CAD build for the part. Positions are in the model's coordinates, mm. Face numbers are marked on the shaded views. A direction names the side the tool comes from. Give positions to 0.01 mm unless a question says otherwise; leave off trailing zeros. Order: outer loops, then holes, each group sorted by start corner. A loop starts at its lowest first (then second) coordinate and runs counter-clockwise, first axis right, second up.
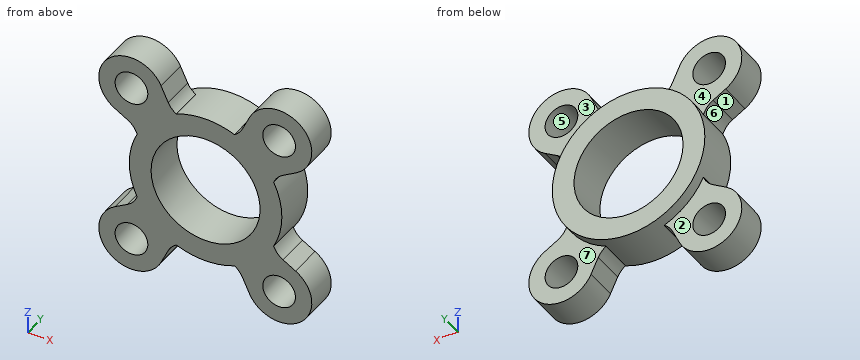
Autodesk Inventor part; units mm, degrees
ref_plane "YZ Plane" through (0, 0, 0) normal (1, 0, 0) x (0, 1, 0)
ref_plane "XZ Plane" through (0, 0, 0) normal (0, 1, 0) x (-1, 0, 0)
ref_plane "XY Plane" through (0, 0, 0) normal (0, 0, 1) x (1, 0, 0)
sketch "Эскиз1" plane through (0, 0, 0) normal (0, 1, 0) x (-1, 0, 0)
  circle A0 centre (-0.0254, 0) radius 7
  circle A1 centre (-7.0254, 6.889) radius 1.5
  circle A2 centre (6.7752, 7.433) radius 1.5
  circle A3 centre (6.9746, -7.0215) radius 1.5
  circle A4 centre (-7.0254, -7.0215) radius 1.5
  circle A5 centre (-0.0254, 0) radius 5
  line L0 (0, 0) -> (0, 8.1981) construction
  line L1 (-0.0254, 0) -> (8.1589, 0) construction
  circle A6 centre (6.7752, 7.433) radius 3
  line L2 (4.0592, 8.7071) -> (3.4025, 7.3072)
  line L3 (8.2851, 4.8407) -> (7.1407, 4.1741)
  line L4 (0.7424, 6.346) -> (0.4551, 6.4808)
  arc A7 (0.7424, 6.346) -> (3.4025, 7.3072) centre (1.5918, 8.1566) ccw
  line L5 (5.7914, 2.5169) -> (6.4192, 1.4392)
  arc A8 (7.1407, 4.1741) -> (6.4192, 1.4392) centre (8.1474, 2.4459) ccw
  point P0 (-10.336, -7.0215)
  point P1 (-9.1433, 6.8618)
  point P2 (6.9746, 10.1261)
  point P3 (2.6587, 6.4649)
  point P4 (6.2546, 3.0921)
  dimension "d0" = 14
  dimension "d1" = 3
  dimension "d2" = 3
  dimension "d3" = 3
  dimension "d4" = 3
  dimension "d5" = 10
  dimension "d6" = 6
  dimension "d7" = 2
  dimension "d8" = 2
extrude "Выдавливание1" add sketch "Эскиз1" along normal blind 4 contours A0
extrude "Выдавливание2" add sketch "Эскиз1" along normal blind 3 contours A0 A7 L2 A6 L3 A8 | A6
mirror "Зеркальное отражение1" about plane through (0, 0, 0) normal (1, 0, 0) of "Выдавливание2"
mirror "Зеркальное отражение2" about plane through (0, 0, 0) normal (0, 0, 1) of "Выдавливание2", "Зеркальное отражение1"
properties part number "крепление подшипника_1"
1. Saw through at B-B on x = 5.75. Give the cut face in (y, z).
2. Saw through at C-C on y = 2.45. State how many separate pieces and enclosed holes the cut face has, plus the area to 3 significant figures.
3. Saw through at D-D on x = -3. Give the cut face in (y, z), plus the area to 3 significant figures.
4. Pin check, flat tips, straight feed: P1, Ø1.5, axis at y = 1.5, z = 4.5, coming from the -X side; P2, Ø5, axis at x = 6.78, z = -7.43, coming from the +Y side; P3, Ø1, axis at y = 3, z = -1.5, coming from the +X side. Stop position of each tip, or through.
5. Mould opens along X. For the marked faces 5, 6 and 7 say: released by +X, released by -X, zero draft, split by the parting line, or undercut.
6. Saw through at A-A on z = 0. Give the cut face in (x, y), plus the area to 3 significant figures.
7. 3-axis set-ups, long thin cutter, end or side, ignore diameter. For the marked faces 1, 2, 3 and 4: which of +Z, -Z, +X, -X, +Y, -Y reach the whole face in a straight line?
8. Wall check: line 1 (Z direction, x = 0, y = 2.85); line 2 (X direction, y = 2.15, z = 8.25); line 3 (Z direction, x = 8, y = 0.3). Give the ranges that are in metal, low to high.
Reported:
1. outline: (0, -10.25) - (3, -10.25) - (3, -8.53) - (0, -8.53) - close; (0, -6.34) - (3, -6.34) - (3, -4.03) - (4, -4.03) - (4, 4.03) - (3, 4.03) - (3, 6.34) - (0, 6.34) - close; (0, 8.53) - (3, 8.53) - (3, 10.25) - (0, 10.25) - close
2. separate pieces: 1
2. enclosed holes: 5
2. area: 172 mm2
3. outline: (0, -6.74) - (3, -6.74) - (3, -6.31) - (4, -6.31) - (4, -3.98) - (0, -3.98) - close; (0, 3.98) - (4, 3.98) - (4, 6.31) - (3, 6.31) - (3, 6.74) - (0, 6.74) - close
3. area: 21.2 mm2
4. P1: stops at x = -8.83
4. P2: stops at y = 3
4. P3: stops at x = 6.95
5. face 5: undercut
5. face 6: released by -X
5. face 7: zero draft
6. outline: (-6.97, 0) - (-4.97, 0) - (-4.97, 4) - (-6.97, 4) - close; (5.03, 0) - (7.03, 0) - (7.03, 4) - (5.03, 4) - close
6. area: 16.0 mm2
7. face 1: -X, +Y, -Y
7. face 2: -Z, -X, +Y
7. face 3: +Z, +X, +Y
7. face 4: +Z, -X, +Y
8. line 1: z = -7 to -5, 5 to 7
8. line 2: x = -9.66 to -8.03, -5.52 to -3.84, 3.84 to 5.52, 8.03 to 9.66
8. line 3: z = -10.17 to -8.3, -6.57 to -4.67, 4.67 to 6.57, 8.3 to 10.17
